Input: part model. Units: mm. Frame: model coordinates. Face numbers are marked on the shaded views. A direction names the side the tool comes from. Round coordinates to 2 decimals unless told otherwise and drop trailing zeros. Loops run counter-clockwise (first coordinate to the right, second up) from the corner with the lowest first, then second, coordinate; pieces in that order, holes last. Notation, with made-up numbers: (-26, 2) -> (-15, 2) arc R11 cw to (-15, 23) -> close; hole circle Ø8 at (76.5, -39). An arc over 180 degrees is marked (long way). Answer in a Markdown table with one row per item. Add a question column.
Q1. Reachability of the marked faces 4 and 5 from +Z, -Z, +X, -X, +Y, -Y: full face, straight path, thin tool, end or side. Return the list, or none.
Q2. Mould query, pull axis Z, two halves, no side actions, for the marked faces 1, 2 and 3. Classes: pulls with the +Z half, pulls with the -Z half, needs draft (parallel to the pull), parting line crosses it, or undercut.
Q3. Pin query (flat end, axial travel): pin 1 (3 mm diameter, centred on y = 2.5, z = -0.5, fed in from +X); pin 2 (10 mm diameter, centred on x = -2.5, z = -4, fed in from -Y); pin 3 (3 mm diameter, centred on x = 0, y = 3.5, fed in from -Z). Return the tip coordinate at first contact, or that it passes through.
Q4. Ray query, L1, parallel to Z at x = 2.5, y = 1.5; L2, parallel to Y at x = -5.25, z = -0.5; L3, parallel to X at y = 2.75, z = -2. Return the intervals inside material, ascending. Write a range as from..to.
Q5. Section A-A, the plane y = 4.25. Output: boundary loops of the cut face in (x, z), and give its area (3 significant figures).
```python
from build123d import *

# Parameters (mm, degrees)
SKETCH2_W           = 6.4262
SKETCH2_H           = 6.4262
CUT_EXTRUDE1_DEPTH  = 6.715
DRAFT1_ANGLE        = 1
BOSS_EXTRUDE2_DEPTH = 2.54
BOSS_EXTRUDE2_TAPER = 1
BOSS_EXTRUDE3_DEPTH = 0.508
BOSS_EXTRUDE3_TAPER = 1
CUT_EXTRUDE2_DEPTH  = 6.5372
CUT_EXTRUDE2_TAPER  = 1


with BuildPart() as part:
    # Sketch1 → Revolve1 (revolve)
    with BuildSketch(Plane.XY):
        Polygon((0, 0), (9.525, 0), (9.525, 2.9972), (6.2865, 2.9972), (6.2865, 6.223), (0, 6.223), align=None)
    revolve(axis=Axis((0, -4.12115, 0), (0, 1, 0)))

    # Sketch2 → Cut-Extrude1 (cut, through all)
    with BuildSketch(Plane(origin=(0, 0.508, 0), x_dir=(1, 0, 0), z_dir=(0, 1, 0))):
        Rectangle(SKETCH2_W, SKETCH2_H)
    extrude(amount=CUT_EXTRUDE1_DEPTH, mode=Mode.SUBTRACT)

    # Sketch3 → Cut-Revolve1 (revolve, cut)
    with BuildSketch(Plane.XY):
        Polygon((0, 6.223), (4.699, 6.223), (0, 1.524), align=None)
    revolve(axis=Axis((0, 0, 0), (0, 1, 0)), mode=Mode.SUBTRACT)

    # Draft1
    draft1_faces = [part.faces().sort_by_distance(p)[0] for p in [
        (-9.525, 1.4986, 0),
    ]]
    draft(draft1_faces, Plane(origin=(9.525, 2.9972, 0), x_dir=(0, 0, 1), z_dir=(0, 1, 0)), DRAFT1_ANGLE)

    # Sketch4 → Boss-Extrude2 (add)
    with BuildSketch(Plane.XZ):
        with BuildLine():
            ThreePointArc((5.337752, -3.855992), (5.351306, -5.763469), (7.181023, -6.302716))
            ThreePointArc((7.181023, -6.302716), (8.233547, -4.861812), (9.000511, -3.250672))
            ThreePointArc((9.000511, -3.250672), (7.655973, -1.897575), (5.971572, -2.792809))
            ThreePointArc((5.971572, -2.792809), (5.679626, -3.339283), (5.337752, -3.855992))
        make_face()
    extrude(amount=BOSS_EXTRUDE2_DEPTH, taper=BOSS_EXTRUDE2_TAPER)

    # Sketch5 → Boss-Extrude3 (add)
    with BuildSketch(Plane.XZ):
        with BuildLine():
            Line((-6.159337, 5.690783), (-7.058911, 6.472771))
            ThreePointArc((-7.058911, 6.472771), (-7.228092, 6.283285), (-7.392189, 6.089379))
            Line((-7.392189, 6.089379), (-6.492615, 5.307391))
            Line((-6.492615, 5.307391), (-6.159337, 5.690783))
        make_face()
    extrude(amount=BOSS_EXTRUDE3_DEPTH, taper=BOSS_EXTRUDE3_TAPER)

    # Sketch6 → Cut-Extrude2 (cut, through all)
    with BuildSketch(Plane(origin=(0, 2.9972, 0), x_dir=(1, 0, 0), z_dir=(0, 1, 0))):
        with BuildLine():
            Line((-5.08, 8.798818), (-4.699, 8.138907))
            ThreePointArc((-4.699, 8.138907), (0, 9.398), (4.699, 8.138907))
            Line((4.699, 8.138907), (5.08, 8.798818))
            ThreePointArc((5.08, 8.798818), (0, 10.16), (-5.08, 8.798818))
        make_face()
    extrude(amount=-CUT_EXTRUDE2_DEPTH, taper=CUT_EXTRUDE2_TAPER, mode=Mode.SUBTRACT)


solid = part.part
```
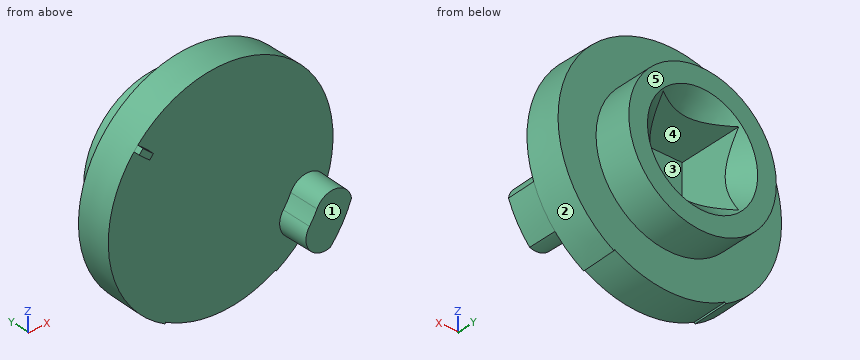
Answer block:
| question | item | result |
|---|---|---|
| 1 | face 4 | +Y |
| 1 | face 5 | +Z, -Z, +X, -X, +Y |
| 2 | face 1 | needs draft |
| 2 | face 2 | parting line crosses it |
| 2 | face 3 | undercut |
| 3 | pin 1 | x = 9.56 |
| 3 | pin 2 | y = 0 |
| 3 | pin 3 | z = -9.42 |
| 4 | L1 | -9.09..-3.21, 3.21..9.22 |
| 4 | L2 | 0..6.22 |
| 4 | L3 | -9.32..-3.21, 3.21..9.32 |
| 5 | outline | circle Ø12.57 at (0, 0); hole (-3.21, -3.21) -> (3.21, -3.21) -> (3.21, 3.21) -> (-3.21, 3.21) -> close |
| 5 | area | 82.9 mm^2 |
